Read the model definition and answer for the solid it produces. Units are mm, in the model's axes. A direction names the side the tool comes from. Round coordinates to 2 decimals unless told otherwise and drop trailing zeros. Order: outer loops, then holes, each group sorted by start corner. A loop starts at its lowest first (then second) coordinate and runs counter-clockwise, first axis right, second up. Notation, with made-up numbers: (-5.75, 83) -> (44.25, 83) arc R25 cw to (44.25, 119) -> close; hole circle Ø2 at (62, 24.5). An arc over 180 degrees is marked (long way). Answer as a JSON object with one key per item and string values. Group by question number.
Item 1: Consider probe 1 along X at (y, z) = (7.25, -63.5); probe 2 along Z at (x, y) = (42, 7.5); probe 3 along Z at (x, y) = (82.55, 8.5). Determine where each line is inside the solid, lowest interval first. Write a range as from..to.
Item 2: Section D-D, the plane y = 7.5 is taken. Write down the section's boundary in (x, z), plus the area to 3 significant figures.
Item 3: Section A-A, the plane x = 82.55 is taken. Write down the section's boundary in (y, z), plus the area to 3 significant figures.
Item 4: For faces 1 (the flat face through (101.6, 6, -88)), 2 (the flat face through (51, 6, -25.4)), determine the directions among +Z, -Z, +X, -X, +Y, -Y from which every point of the face is accessible in a straight line to the end or side of a thin tool.
Item 5: Section C-C, the plane x = 35.5 is taken. Write down the section's boundary in (y, z), plus the area to 3 significant figures.
Item 6: The mould has two halves that part along Z. Classify faces 3 (the cylindrical face through (21.889, 6.261, -62.023)), 4 (the flat face through (52, 6, -177.8)), 5 (the flat face through (52, 12.7, -88)): pulls with the +Z half, pulls with the -Z half, needs draft (parallel to the pull), parting line crosses it, or undercut.
Item 7: Section B-B, the plane z = -63.5 is taken. Write down the section's boundary in (x, y), plus the area to 3 significant figures.
Autodesk Inventor part; units mm, degrees
ref_plane "YZ Plane" through (0, 0, 0) normal (1, 0, 0) x (0, 1, 0)
ref_plane "XZ Plane" through (0, 0, 0) normal (0, 1, 0) x (-1, 0, 0)
ref_plane "XY Plane" through (0, 0, 0) normal (0, 0, 1) x (1, 0, 0)
sketch "Sketch1" plane through (0, 0, 0) normal (0, 1, 0) x (-1, 0, 0)
  point P0 (0, 0)
sketch "Sketch2" plane through (0, 0, 0) normal (0, 1, 0) x (-1, 0, 0)
  point P0 (0, 0)
sketch "Sketch3" plane through (0, 0, 0) normal (0, 1, 0) x (-1, 0, 0)
  point P0 (0, 0)
sketch "Sketch4" plane through (0, 0, 0) normal (0, 1, 0) x (-1, 0, 0)
  line L0 (0, 0) -> (-101.6, 0)
  line L1 (-101.6, 0) -> (-101.6, -177.8)
  line L2 (-101.6, -177.8) -> (0, -177.8)
  line L3 (0, -177.8) -> (0, 0)
  line L4 (-50.8, -25.4) -> (-69.85, -25.4)
  line L5 (-69.85, -25.4) -> (-31.75, -25.4)
  line L6 (-31.75, -25.4) -> (-31.75, -38.1)
  line L7 (-31.75, -38.1) -> (-69.85, -38.1)
  line L8 (-69.85, -38.1) -> (-69.85, -25.4)
  line L9 (-50.8, -177.8) -> (-50.8, -152.4)
  line L10 (-50.8, -152.4) -> (-31.75, -152.4)
  line L11 (-31.75, -152.4) -> (-31.75, -139.7)
  line L12 (-31.75, -139.7) -> (-69.85, -139.7)
  line L13 (-69.85, -139.7) -> (-69.85, -152.4)
  line L14 (-69.85, -152.4) -> (-50.8, -152.4)
  dimension "d0" = 101.6
  dimension "d1" = 177.8
  dimension "d3" = 19.05
  dimension "d4" = 38.1
  dimension "d5" = 12.7
  dimension "d6" = 38.1
  dimension "d7" = 25.4
  dimension "d8" = 19.05
  dimension "d9" = 12.7
  dimension "d10" = 38.1
  dimension "d11" = 12.7
extrude "Extrusion1" add sketch "Sketch4" along normal blind 12.7
sketch "Sketch5" plane through (0, 12.7, 0) normal (0, 1, 0) x (1, 0, 0)
  circle A0 centre (19.05, 63.5) radius 3.9688
  circle A1 centre (82.55, 63.5) radius 3.9687
  point P0 (0, 0)
  point P1 (31.75, 38.1)
  dimension "d19" = 7.9375
  dimension "d21" = 7.9375
hole "Hole1" at (19.05, 12.7, -63.5) direction (0, -1, 0) diameter 6.4008 end through all
hole "Hole2" at (82.55, 12.7, -63.5) direction (0, -1, 0) diameter 6.4008 end through all
equation "\"d23\" = d12"
equation "\"d30\" = d12"
properties part number "wrist_plate"
Values found:
{
 "1": {"probe 1": "0..15.85, 22.25..79.35, 85.75..101.6", "probe 2": "-177.8..-152.4, -139.7..-38.1, -25.4..0", "probe 3": "-177.8..-66.7, -60.3..0"},
 "2": {"outline": "(0, -177.8) -> (101.6, -177.8) -> (101.6, 0) -> (0, 0) -> close; hole circle Ø6.4 at (19.05, -63.5); hole (31.75, -152.4) -> (69.85, -152.4) -> (69.85, -139.7) -> (31.75, -139.7) -> close; hole (31.75, -38.1) -> (69.85, -38.1) -> (69.85, -25.4) -> (31.75, -25.4) -> close; hole circle Ø6.4 at (82.55, -63.5)", "area": "17,000 mm2"},
 "3": {"outline": "(0, -177.8) -> (12.7, -177.8) -> (12.7, -66.7) -> (0, -66.7) -> close; (0, -60.3) -> (12.7, -60.3) -> (12.7, 0) -> (0, 0) -> close", "area": "2,180 mm2"},
 "4": {"face 1": "+Z, -Z, +X, +Y, -Y", "face 2": "+Y, -Y"},
 "5": {"outline": "(0, -177.8) -> (12.7, -177.8) -> (12.7, -152.4) -> (0, -152.4) -> close; (0, -139.7) -> (12.7, -139.7) -> (12.7, -38.1) -> (0, -38.1) -> close; (0, -25.4) -> (12.7, -25.4) -> (12.7, 0) -> (0, 0) -> close", "area": "1,940 mm2"},
 "6": {"face 3": "undercut", "face 4": "pulls with the -Z half", "face 5": "needs draft"},
 "7": {"outline": "(0, 0) -> (15.85, 0) -> (15.85, 12.7) -> (0, 12.7) -> close; (22.25, 0) -> (79.35, 0) -> (79.35, 12.7) -> (22.25, 12.7) -> close; (85.75, 0) -> (101.6, 0) -> (101.6, 12.7) -> (85.75, 12.7) -> close", "area": "1,130 mm2"}
}
